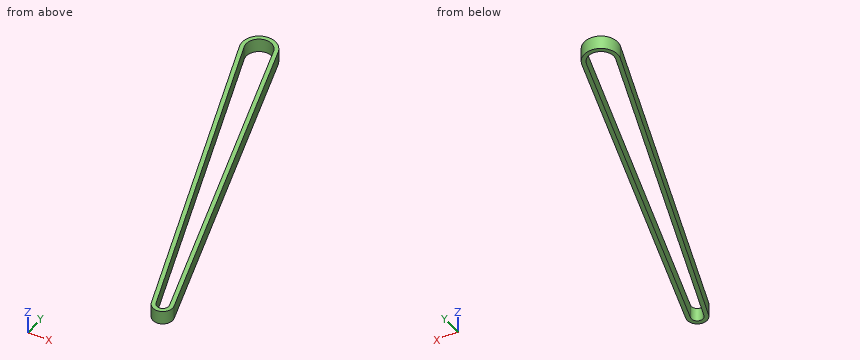
Autodesk Inventor part; units mm, degrees
ref_plane "YZ Plane" through (0, 0, 0) normal (1, 0, 0) x (0, 1, 0)
ref_plane "XZ Plane" through (0, 0, 0) normal (0, 1, 0) x (-1, 0, 0)
ref_plane "XY Plane" through (0, 0, 0) normal (0, 0, 1) x (1, 0, 0)
sketch "Sketch1" plane through (0, 0, 0) normal (0, 0, 1) x (1, 0, 0)
  circle A0 centre (0, 0) radius 4.7625 construction
  circle A1 centre (37.9719, -120.3156) radius 2.1844 construction
  arc A2 (35.9027, -121.0155) -> (40.068, -119.7009) centre (37.9719, -120.3156) ccw
  arc A3 (4.57, 1.3403) -> (-4.5114, -1.5259) centre (0, 0) ccw
  line L0 (-4.5114, -1.5259) -> (35.9027, -121.0155)
  line L1 (40.068, -119.7009) -> (4.57, 1.3403)
  line L2 (34.4817, -121.4961) -> (-5.9324, -2.0065)
  arc A4 (6.0094, 1.7624) -> (-5.9324, -2.0065) centre (0, 0) ccw
  line L3 (6.0094, 1.7624) -> (41.5074, -119.2787)
  arc A5 (34.4817, -121.4961) -> (41.5074, -119.2787) centre (37.9719, -120.3156) ccw
  point P0 (0, 0)
  dimension "d0" = 4.3688
  dimension "d1" = 1.5
extrude "Extrusion1" add sketch "Sketch1" along normal blind 5 and the other way blind 5
sketch "Sketch2" plane through (34.4817, -121.4961, -5) normal (-0.9473, -0.3204, 0) x (0, 0, 1)
  line L0 (0, 132.4016) -> (10, 132.4016)
  line L1 (10, 126.1391) -> (10, 0)
  line L2 (0, 0) -> (0, 126.1391)
  line L3 (0, -3.6844) -> (10, -3.6844)
  line L4 (0, 0) -> (0, -3.6844)
  line L5 (0, 0) -> (0, -3.6844)
  line L6 (10, -3.6844) -> (10, 0)
  line L7 (10, -3.6844) -> (10, 0)
  line L8 (10, 132.4016) -> (10, 126.1391)
  line L9 (10, 125.8832) -> (10, 132.4016)
  line L10 (0, 132.4016) -> (0, 126.1391)
  line L11 (0, 132.4016) -> (0, 125.8832)
  line L12 (5, -3.6844) -> (10, 132.4016)
  line L13 (0, -3.6844) -> (5, 132.4016)
  point P0 (5, 126.1391)
  point P1 (0, -0.1505)
  point P2 (10, -0.1505)
  dimension "d6" = 5
  dimension "d7" = 5
extrude "Extrusion2" cut sketch "Sketch2" against normal blind 25.4 contours L0 L13 L4 L2 L10 | L8 L1 L6 L3 L12
properties part number "Angle Changer right band"
Verification items for the finished model (mm, model axes). Round coordinates to 2 decimals unless told otherwise and drop trailing zeros. Order: outer loops, then holes, each group sorted by start corner. A loop starts at its lowest first (then second) coordinate and runs counter-clockwise, first axis right, second up. Notation, with made-up numbers: (67, 52.5) - (105, 52.5) arc R6 ccw to (105, 62.5) - close; hole circle Ø5 at (45, 7). An arc over 180 degrees is marked (long way). Use CSV: the item, a comma, the result in double quotes. Start each with the question number.
1) Section check A-A, the plane x = 30.5. Record the cut outline in (y, z).
2) Section check B-B, the plane y = -23.5. Record the cut outline in (x, z).
3) Go/stop test with flat-tipped pins: P1, Ø2, axis at y = -104.5, z = -3, coming from the -X side (3 decimals); P2, Ø3, axis at x = 33.5, y = -83, coming from the -Z side; P3, Ø3, axis at x = 20, y = -73, coming from the +Z side; P4, Ø8, axis at x = 5, y = -9, coming from the -Z side. Record where each tip stops, or that it passes through.
4) Thickness scan on L1, parallel to X at y = -86, z = 1; L2, parallel to X at y = -78.5, z = 1.5; L3, parallel to Z at x = 13.5, y = -58. Record the ranges inside material, lowest first.
5) Section check C-C, the plane z = -2. Record the cut outline in (x, y).
Answers:
1,outline,"(-109.72, -4.41) - (-105.04, -4.25) - (-105.04, 0.75) - (-109.72, 0.59) - close; (-87.08, -3.62) - (-81.75, -3.43) - (-81.75, 1.57) - (-87.08, 1.38) - close"
2,outline,"(1.34, -1.06) - (2.92, -1.08) - (2.92, 3.92) - (1.34, 3.94) - close; (11.85, -1.19) - (13.42, -1.21) - (13.42, 3.79) - (11.85, 3.81) - close"
3,P1,"stops at x = 28.395"
3,P2,"passes through"
3,P3,"stops at z = 2.05"
3,P4,"stops at z = -0.72"
4,L1,"x = 22.48 to 24.06, 30.18 to 31.75"
4,L2,"x = 19.94 to 21.52, 27.98 to 29.55"
4,L3,"z = -2.41 to 2.59"
5,outline,"(9.5, -47.64) - (34.48, -121.5) arc R3.68 ccw to (41.51, -119.28) - (19.51, -44.26) - (18.08, -44.74) - (40.07, -119.7) arc R2.18 cw to (35.9, -121.02) - (10.92, -47.16) - close"
